from build123d import *

# Parameters (mm, degrees)
SKETCH2_W                                       = 117
SKETCH2_H                                       = 135
BOSS_EXTRUDE1_DEPTH                             = 10
SKETCH4_W                                       = 107
SKETCH4_H                                       = 107
CUT_EXTRUDE1_DEPTH                              = 5
SKETCH3_R                                       = 1.75
CUT_EXTRUDE2_DEPTH                              = 90.462282555
CSK_FOR_M6_FLAT_HEAD_MACHINE_SCREW1_D           = 7
CSK_FOR_M6_FLAT_HEAD_MACHINE_SCREW1_CSINK_D     = 12.6
CSK_FOR_M6_FLAT_HEAD_MACHINE_SCREW1_CSINK_ANGLE = 90
FILLET1_R                                       = 20
FILLET2_R                                       = 2


with BuildPart() as part:
    # Sketch2 → Boss-Extrude1 (new body)
    with BuildSketch(Plane(origin=(0, 0, 0), x_dir=(1, 0, 0), z_dir=(0, 1, 0))):
        Rectangle(SKETCH2_W, SKETCH2_H)
    extrude(amount=BOSS_EXTRUDE1_DEPTH)

    # Sketch4 → Cut-Extrude1 (cut)
    with BuildSketch(Plane(origin=(0, 10, 0), x_dir=(1, 0, 0), z_dir=(0, 1, 0))):
        with Locations((0, -9)):
            Rectangle(SKETCH4_W, SKETCH4_H)
    extrude(amount=-CUT_EXTRUDE1_DEPTH, mode=Mode.SUBTRACT)

    # Sketch3 → Cut-Extrude2 (cut, through all)
    with BuildSketch(Plane(origin=(0, 5, 0), x_dir=(1, 0, 0), z_dir=(0, 1, 0))):
        with Locations(Location((-31.5, 37, 0), (0, 0, 270))):
            Circle(SKETCH3_R)
        with Locations(Location((47, 37, 0), (0, 0, 270))):
            Circle(SKETCH3_R)
        with Locations(Location((47, -55, 0), (0, 0, 270))):
            Circle(SKETCH3_R)
        with Locations(Location((-31.5, -55, 0), (0, 0, 270))):
            Circle(SKETCH3_R)
    extrude(amount=-CUT_EXTRUDE2_DEPTH, mode=Mode.SUBTRACT)

    # CSK for M6 Flat Head Machine Screw1 (through all)
    with Locations(Plane(origin=(0, 10, 0), x_dir=(1, 0, 0), z_dir=(0, 1, 0))):
        with Locations((-15, 56), (15, 56)):
            CounterSinkHole(CSK_FOR_M6_FLAT_HEAD_MACHINE_SCREW1_D / 2, CSK_FOR_M6_FLAT_HEAD_MACHINE_SCREW1_CSINK_D / 2, counter_sink_angle=CSK_FOR_M6_FLAT_HEAD_MACHINE_SCREW1_CSINK_ANGLE)

    # Fillet1
    fillet1_edges = [part.edges().sort_by_distance(p)[0] for p in [
        (-58.5, 5, -67.5),
        (58.5, 5, -67.5),
    ]]
    fillet(fillet1_edges, radius=FILLET1_R)

    # Fillet2
    fillet2_edges = [part.edges().sort_by_distance(p)[0] for p in [
        (0, 10, 67.5),
        (58.5, 10, 10),
        (0, 10, -67.5),
        (-58.5, 10, 10),
        (-52.642135624, 10, -61.642135624),
        (52.642135624, 10, -61.642135624),
    ]]
    fillet(fillet2_edges, radius=FILLET2_R)


solid = part.part
Read the model definition and answer for the solid it produces. Units are mm, in the model's axes. A direction names the side the tool comes from. Give positions to 0.01 mm unless a question says otherwise; leave off trailing zeros. Loops run counter-clockwise (first coordinate to the right, second up) from the corner with the lowest first, then second, coordinate; pieces in that order, holes last. Notation, with made-up numbers: (64.25, 35) -> (92.25, 35) arc R22 cw to (92.25, 57) -> close; hole circle Ø1 at (42.25, 69). An arc over 180 degrees is marked (long way). Use a Markdown table: item, result.
Q1. Section D-D, the plane z = 0 is taken. Determine the outline of the cut face in (x, y), then the cut area to 3 significant figures.
Solved:
| item | result |
|---|---|
| outline | (-58.5, 0) -> (58.5, 0) -> (58.5, 8) arc R2 ccw to (56.5, 10) -> (53.5, 10) -> (53.5, 5) -> (-53.5, 5) -> (-53.5, 10) -> (-56.5, 10) arc R2 ccw to (-58.5, 8) -> close |
| area | 633 mm^2 |
Q2. Each of these flat-tipped pins is pushed along its axis until it touches: pin 1 (3 mm diameter, centred on x = -31.5, z = 55, fed in from +Y); pin 2 (9 mm diameter, centred on x = -15, z = -56, fed in from +Y); pin 3 (5.5 mm diameter, centred on x = 47, z = 55, fed in from +Y); pin 4 (11 mm diameter, centred on x = 15, z = -56, fed in from +Y). Where does it stop, or does it pass through?
Solved:
| item | result |
|---|---|
| pin 1 | passes through |
| pin 2 | stops at y = 8.2 |
| pin 3 | stops at y = 5 |
| pin 4 | stops at y = 9.2 |
Q3. A tool of negligible diameter and unlimited length cuts with its end or side. For faces 1 (the face through (-1, 0, -1)), 2 (the face through (-1, 5, 8)), from which of +Z, -Z, +X, -X, +Y, -Y can it reach the whole face along a straight path? Write none if from no direction.
Solved:
| item | result |
|---|---|
| face 1 | +Z, -Z, +X, -X, -Y |
| face 2 | +Y |
Q4. Determine the mould class of faces 3 (the face through (-58.5, 4, 11)), 4 (the face through (45.45, 2.54, -36.19)), 5 (the face through (58.5, 4, 11)), 6 (the face through (13.32, 7.34, -52.77)) for opening direction X: pulls with the +X half, pulls with the -X half, needs draft (parallel to the pull), parting line crosses it, or undercut.
Solved:
| item | result |
|---|---|
| face 3 | pulls with the -X half |
| face 4 | undercut |
| face 5 | pulls with the +X half |
| face 6 | undercut |
Q5. Section C-C, the plane x = 15 is taken. Determine the outline of the cut face in (y, z), then the cut area to 3 significant figures.
Solved:
| item | result |
|---|---|
| outline | (0, -67.5) -> (8, -67.5) arc R2 ccw to (10, -65.5) -> (10, -62.3) -> (7.2, -59.5) -> (0, -59.5) -> close; (0, -52.5) -> (7.2, -52.5) -> (10, -49.7) -> (10, -44.5) -> (5, -44.5) -> (5, 62.5) -> (10, 62.5) -> (10, 65.5) arc R2 ccw to (8, 67.5) -> (0, 67.5) -> close |
| area | 735 mm^2 |
Q6. Find the intervals of material crossed by line 1 along X through (y, z) = (3.85, 55); line 2 along X through (y, z) = (6.25, -5); line 3 along Z through (x, y) = (-24, 5.25), in increasing order.
Solved:
| item | result |
|---|---|
| line 1 | x = -58.5 to -33.25, -29.75 to 45.25, 48.75 to 58.5 |
| line 2 | x = -58.5 to -53.5, 53.5 to 58.5 |
| line 3 | z = -67.5 to -44.5, 62.5 to 67.5 |
Q7. Section A-A, the plane z = 55 is taken. Determine the outline of the cut face in (x, y).
Solved:
| item | result |
|---|---|
| outline | (-58.5, 0) -> (-33.25, 0) -> (-33.25, 5) -> (-53.5, 5) -> (-53.5, 10) -> (-56.5, 10) arc R2 ccw to (-58.5, 8) -> close; (-29.75, 0) -> (45.25, 0) -> (45.25, 5) -> (-29.75, 5) -> close; (48.75, 0) -> (58.5, 0) -> (58.5, 8) arc R2 ccw to (56.5, 10) -> (53.5, 10) -> (53.5, 5) -> (48.75, 5) -> close |
Q8. Section B-B, the plane x = -31.5 is taken. Determine the outline of the cut face in (y, z).
Solved:
| item | result |
|---|---|
| outline | (0, -67.5) -> (8, -67.5) arc R2 ccw to (10, -65.5) -> (10, -44.5) -> (5, -44.5) -> (5, -38.75) -> (0, -38.75) -> close; (0, -35.25) -> (5, -35.25) -> (5, 53.25) -> (0, 53.25) -> close; (0, 56.75) -> (5, 56.75) -> (5, 62.5) -> (10, 62.5) -> (10, 65.5) arc R2 ccw to (8, 67.5) -> (0, 67.5) -> close |
